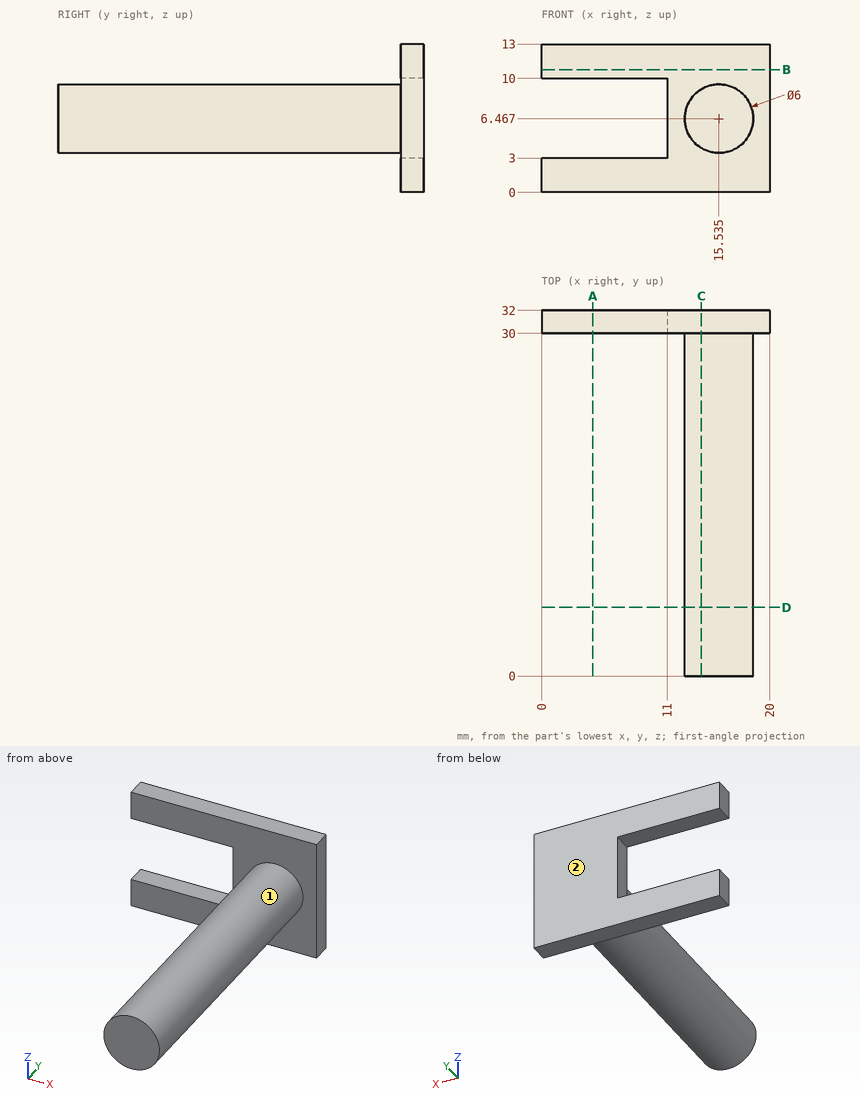
Could you check a few things on this drawing? It's one solid part, dimensions in mm from its lowest x, y, z. A direction names the side the tool comes from. Give positions to 0.01 mm unless a question says otherwise; leave off trailing zeros. Order: outer loops, then holes, each group sorted by start corner. A loop starts at its lowest first (then second) coordinate and runs counter-clockwise, first axis right, second up. Notation, with made-up numbers: (67, 66) -> (103, 66) arc R7 ccw to (103, 71) -> close; hole circle Ø9 at (-1.75, 0). An arc over 180 degrees is marked (long way). Use CSV: the item, a comma, the result in double quotes. Start each with the question number.
Item 1: If I drill on probe 1 along Y at (x, z) = (17, 10.5); probe 2 along Z at (x, y) = (15.5, 29); probe 3 along X at (y, z) = (8, 6.25), over which ranges is the centre line in solid material (lowest first)? Write a range as [from, to].
Item 2: I'm going to push flat-ended pins straight in: P1, Ø12, axis at x = 10.5, y = 14.5, coming from the +Z side; P2, Ø6.5, axis at x = 6.5, z = 4, coming from the -Y side; P3, Ø2, axis at y = 31, z = 7.5, coming from the -X side. Where does each tip first touch, or does it pass through?
Item 3: Suppose I cut it at A-A (x = 4.5). List the corners of the cut face in (y, z) for me, and give its area (3 significant figures).
Item 4: Suppose I cut it at D-D (y = 6). List the corners of the cut face in (x, z) for me (1 decimal).
Item 5: Suppose I cut it at B-B (z = 10.75). List the corners of the cut face in (x, y) for me, and give its area (3 significant figures).
Item 6: On a 3-axis mill with a long thin cutter (end or side, diameter ignored), from which of +Z, -Z, +X, -X, +Y, -Y can I reach the whole of each face in a straight line? I mean the marked faces 1 and 2. Say none if no direction works.
Item 7: Suppose I cut it at C-C (x = 14). List the corners of the cut face in (y, z) for me.
Answer block:
1,probe 1,"y = [30, 32]"
1,probe 2,"z = [3.47, 9.47]"
1,probe 3,"x = [12.54, 18.53]"
2,P1,"stops at z = 9.47"
2,P2,"stops at y = 30"
2,P3,"stops at x = 11"
3,outline,"(30, 0) -> (32, 0) -> (32, 3) -> (30, 3) -> close; (30, 10) -> (32, 10) -> (32, 13) -> (30, 13) -> close"
3,area,"12.0 mm^2"
4,outline,"circle Ø6 at (15.5, 6.5)"
5,outline,"(0, 30) -> (20, 30) -> (20, 32) -> (0, 32) -> close"
5,area,"40.0 mm^2"
6,face 1,"-Y"
6,face 2,"+Z, -Z, +X, -X, +Y"
7,outline,"(0, 3.89) -> (30, 3.89) -> (30, 0) -> (32, 0) -> (32, 13) -> (30, 13) -> (30, 9.04) -> (0, 9.04) -> close"
